Check sheet for the modelled part. Datum: model origin and axes. Units: mm. Face numbers are marked on the shaded views. Give positions to 0.01 mm unless a question says otherwise; leave off trailing zeros. Order: outer loops, then holes, each group sorted by start corner. A loop starts at its lowest first (then second) coordinate and runs counter-clockwise, first axis right, second up.
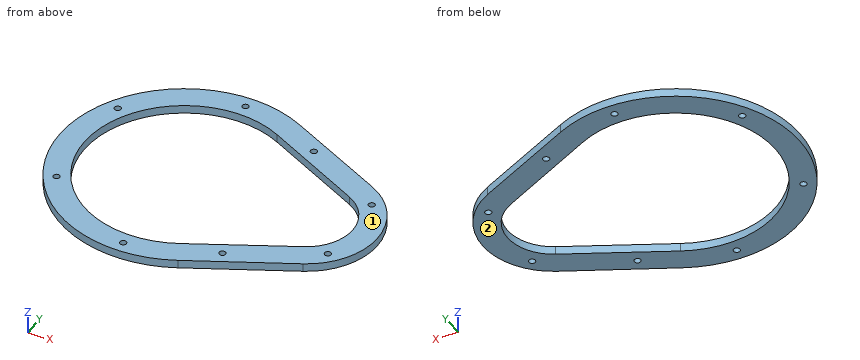
```python
from build123d import *

# Parameters (mm, degrees)
BOSS_EXTRUDE2_DEPTH     = 4
CUT_EXTRUDE4_DEPTH      = 6
CUT_EXTRUDE4_DEPTH_BACK = 111.961995243
SKETCH11_R              = 1.55


with BuildPart() as part:
    # Sketch1 → Boss-Extrude2 (new body)
    with BuildSketch(Plane.XY):
        with BuildLine():
            Line((26.280991736, 53.938015104), (74.102766205, 30.637126906))
            ThreePointArc((74.102766205, 30.637126906), (93.255371901, 0), (74.102766205, -30.637126906))
            Line((74.102766205, -30.637126906), (26.280991736, -53.938015104))
            ThreePointArc((26.280991736, -53.938015104), (-60, 0), (26.280991736, 53.938015104))
        make_face()
        with BuildLine():
            Line((21.297534718, 43.26272971), (68.929300346, 19.81439002))
            ThreePointArc((68.929300346, 19.81439002), (81.260208333, 0), (68.929300346, -19.81439002))
            Line((68.929300346, -19.81439002), (21.297534718, -43.26272971))
            ThreePointArc((21.297534718, -43.26272971), (-48.22083333, 0), (21.297534718, 43.26272971))
        make_face(mode=Mode.SUBTRACT)
    extrude(amount=BOSS_EXTRUDE2_DEPTH)

    # Sketch11 → Cut-Extrude4 (cut, two sides: drawn at the far end of the back side and taken through both)
    with BuildSketch(Plane.XY.offset(4).offset(-CUT_EXTRUDE4_DEPTH_BACK)):
        with Locations((0, 54.22083333)):
            Circle(SKETCH11_R)
        with Locations((-46.956619078, 27.110416665)):
            Circle(SKETCH11_R)
        with Locations((-46.956619078, -27.110416665)):
            Circle(SKETCH11_R)
        with Locations((0, -54.22083333)):
            Circle(SKETCH11_R)
        with Locations((79.945436483, 19.445436483)):
            Circle(SKETCH11_R)
        with Locations((40.498188633, 40.498188633)):
            Circle(SKETCH11_R)
        with Locations(Location((79.945436483, -19.445436483, 0), (0, 0, 180))):
            Circle(SKETCH11_R)
        with Locations(Location((40.498188633, -40.498188633, 0), (0, 0, 180))):
            Circle(SKETCH11_R)
    extrude(amount=CUT_EXTRUDE4_DEPTH + CUT_EXTRUDE4_DEPTH_BACK, mode=Mode.SUBTRACT)


solid = part.part
```
(1) Cross-section at A-A on x = -30.5. Enter the section's corners in (y, z), then the cut area to 3 significant figures.
Response values:
outline: (-51.67, 0) - (-37.35, 0) - (-37.35, 4) - (-51.67, 4) - close; (37.35, 0) - (51.67, 0) - (51.67, 4) - (37.35, 4) - close
area: 115 mm2
(2) Cross-section at B-B on y = 0. Enter the section's corners in (x, z).
Response values:
outline: (-60, 0) - (-48.22, 0) - (-48.22, 4) - (-60, 4) - close; (81.26, 0) - (93.26, 0) - (93.26, 4) - (81.26, 4) - close
(3) Cross-section at C-C on z = 2.6. Count the separate pieces of the cut face and the enclosed holes in it, then the cut area to 3 significant figures.
Response values:
separate pieces: 1
enclosed holes: 9
area: 4,540 mm2
(4) Material ranges on L1, parallel to Y at x = 0, z = 3.15; L2, parallel to Y at x = 70.5, z = 1.5; L3, parallel to X at y = -22, z = 2.65, recorded low to high.
Response values:
L1: y = -60 to -55.77, -52.67 to -48.22, 48.22 to 52.67, 55.77 to 60
L2: y = -32.39 to -18.96, 18.96 to 32.39
L3: x = -55.82 to -42.91, 64.49 to 85.2
(5) Release check for a two-part mould opening along Z. For the marked faces 1 and 2 record: released by +Z, released by -Z, zero draft, split by the parting line, or undercut.
Response values:
face 1: released by +Z
face 2: released by -Z
(6) Gauge pin test, flat ends, axial feed: pin 1 Ø3.5 at (x, y) = (79.95, 19.45) entering from -Z; pin 2 Ø2 at (y, z) = (6, 1.5) entering from -X; pin 3 Ø1.9 at (x, y) = (40.5, 40.5) entering from -Z; pin 4 Ø1.5 at (y, z) = (0.5, 3) entering from -X. Record the tip position at first contact, or that the pin passes through.
Response values:
pin 1: stops at z = 0
pin 2: stops at x = -59.79
pin 3: passes through
pin 4: stops at x = -60
